Check sheet for the modelled part. Datum: model origin and axes. Units: mm. Coordinates: 2 decimals unless noted, no trailing zeros. Write each loop counter-clockwise with the first axis right and the second up, starting at its lowest first coordinate (ties: lowest second). Pieces come first, ordered by that corner, then holes. Notation, with made-up numbers: (1.5, 17) -> (38.5, 17) arc R32 ccw to (38.5, 56) -> close; hole circle Ø9 at (65, 63.25). An arc over 180 degrees is marked (long way). One line per item, written item: value. Start each with the question number.
1) Gauge pin test, flat ends, axial feed: P1, Ø1, axis at x = -34, z = 2.5, coming from the +Y side; P2, Ø2, axis at x = -10.5, z = 1, coming from the -Y side; P3, Ø1.5, axis at y = -3.5, z = 1, coming from the +X side. Record the tip position at first contact, or that the pin passes through.
2) Scan lines: line 1 along X through (y, z) = (4.25, 0.6); line 2 along Y through (x, z) = (-39.5, 3.95); line 3 along Z through (x, y) = (-44.5, -3). Record each from-to range of solid material in increasing order. Write a range as [from, to].
3) Sectioned sample at A-A on y = 3.5. Enter the section's corners in (x, z), plus the area to 3 significant figures.
```python
from build123d import *

# Parameters (mm, degrees)
F1_DEPTH = 2.5
F3_DEPTH = 5


with BuildPart() as f1:
    # F0 (on Front) → F1 (new body, symmetric)
    with BuildSketch(Plane.XZ):
        with BuildLine():
            Line((-43.5, 0), (-1.4094070066, 0))
            add(Edge.make_bspline(
                [(-43.5, 4.8), (-39.8710331933, 5.2983873013), (-40.401533246, 4.8974864185), (-1.4094070066, 0)],
                knots=[0.5607612566, 0.5607612566, 0.5607612566, 0.5607612566, 1, 1, 1, 1], degree=3))
            Line((-43.5, 4.8), (-43.5, 0))
        make_face()
        with BuildLine():
            Line((-47.625, 0), (-43.5, 0))
            Line((-43.5, 0), (-43.5, 4.8))
            add(Edge.make_bspline(
                [(-47.625, 4.1), (-46.191734982, 4.3979293395), (-44.6404650354, 4.643373246), (-43.5, 4.8)],
                knots=[0.422722951, 0.422722951, 0.422722951, 0.422722951, 0.5607612566, 0.5607612566, 0.5607612566, 0.5607612566], degree=3))
            Line((-47.625, 4.1), (-47.625, 0))
        make_face()
        with BuildLine():
            Line((-51.75, 0), (-47.625, 0))
            Line((-47.625, 0), (-47.625, 4.1))
            add(Edge.make_bspline(
                [(-51.75, 3.1), (-50.3924722152, 3.446603597), (-49.0685918755, 3.7999240416), (-47.625, 4.1)],
                knots=[0.2836900617, 0.2836900617, 0.2836900617, 0.2836900617, 0.422722951, 0.422722951, 0.422722951, 0.422722951], degree=3))
            Line((-51.75, 3.1), (-51.75, 0))
        make_face()
        with BuildLine():
            Line((-60, 0), (-55.875, 0))
            Line((-55.875, 0), (-55.875, 1.9))
            add(Edge.make_bspline(
                [(-60, 0), (-58.6279008986, 0.6754279552), (-57.2727716722, 1.3762478568), (-55.875, 1.9)],
                knots=[0, 0, 0, 0, 0.14381593, 0.14381593, 0.14381593, 0.14381593], degree=3))
        make_face()
        with BuildLine():
            Line((-55.875, 0), (-51.75, 0))
            Line((-51.75, 0), (-51.75, 3.1))
            add(Edge.make_bspline(
                [(-55.875, 1.9), (-54.5155393398, 2.4093968124), (-53.1157417417, 2.751299218), (-51.75, 3.1)],
                knots=[0.14381593, 0.14381593, 0.14381593, 0.14381593, 0.2836900617, 0.2836900617, 0.2836900617, 0.2836900617], degree=3))
            Line((-55.875, 1.9), (-55.875, 0))
        make_face()
    extrude(amount=F1_DEPTH, both=True)

    # F2 (on Front) → F3 (join, symmetric)
    with BuildSketch(Plane.XZ):
        with BuildLine():
            Line((-56.3516374265, 0), (-48.6134569347, 0))
            add(Edge.make_bspline(
                [(-45.5359602044, 1.7534863618), (-46.4926973174, 1.2011188271), (-47.5249209999, 0.6140901608), (-48.6134569347, 0)],
                knots=[25.5941661656, 25.5941661656, 25.5941661656, 25.5941661656, 27.1611911657, 27.1611911657, 27.1611911657, 27.1611911657], degree=3))
            Line((-45.5359602044, 1.7534863618), (-56.3582745625, 1.7115182598))
            Line((-56.3582745625, 1.7115182598), (-56.3516374265, 0))
        make_face()
        with BuildLine():
            Line((-48.6134569347, 0), (-16.0882583667, 0))
            Line((-16.0882583667, 0), (-16.0882583667, 1.8676822825))
            Line((-16.0882583667, 1.8676822825), (-45.5359602044, 1.7534863618))
            add(Edge.make_bspline(
                [(-45.5359602044, 1.7534863618), (-46.4926973174, 1.2011188271), (-47.5249209999, 0.6140901608), (-48.6134569347, 0)],
                knots=[25.5941661656, 25.5941661656, 25.5941661656, 25.5941661656, 27.1611911657, 27.1611911657, 27.1611911657, 27.1611911657], degree=3))
        make_face()
    extrude(amount=F3_DEPTH, both=True)


solid = f1.part
```
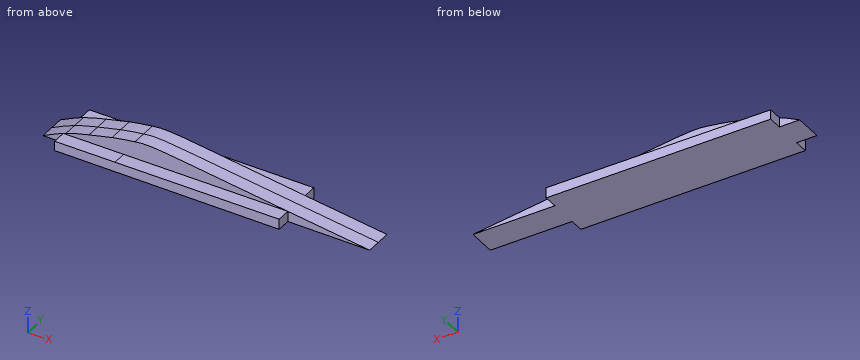
Answers:
1. P1: stops at y = 2.5
1. P2: stops at y = -2.5
1. P3: stops at x = -16.09
2. line 1: x = [-56.35, -16.09]
2. line 2: y = [-2.5, 2.5]
2. line 3: z = [0, 1.76]
3. outline: (-56.36, 1.71) -> (-56.35, 0) -> (-16.09, 0) -> (-16.09, 1.87) -> close
3. area: 72.1 mm2
